from build123d import *

# Parameters (mm, degrees)
F0_W     = 63.5
F0_H     = 63.5
F1_DEPTH = 254
F2_R     = 30.48
F3_W     = 63.5
F3_H     = 33.02
F4_DEPTH = 38.1
F5_R     = 30.48


with BuildPart() as f1:
    # F0 (on Top) → F1 (new body)
    with BuildSketch(Plane.XY):
        with Locations((31.75, 31.75)):
            Rectangle(F0_W, F0_H)
    extrude(amount=F1_DEPTH)

    # F2
    f2_edges = [f1.edges().sort_by_distance(p)[0] for p in [
        (31.75, 0, 254),
    ]]
    fillet(f2_edges, radius=F2_R)

    # F3 (on face) → F4 (join)
    with BuildSketch(Plane.XY.offset(254)):
        with Locations((31.75, 46.99)):
            Rectangle(F3_W, F3_H)
    extrude(amount=F4_DEPTH)

    # F5
    f5_edges = [f1.edges().sort_by_distance(p)[0] for p in [
        (31.75, 63.5, 292.1),
    ]]
    fillet(f5_edges, radius=F5_R)


solid = f1.part
Can you work these out from the model? Positions are in its coordinate system, mm. A direction names the side the tool comes from. Coordinates: 2 decimals unless noted, no trailing zeros. Write each loop counter-clockwise with the first axis right and the second up, starting at its lowest first coordinate (ties: lowest second). Pieces come first, ordered by that corner, then holes. Notation, with made-up numbers: (70.25, 46.5) - (87.25, 46.5) arc R30 ccw to (87.25, 85.5) - close; hole circle Ø10 at (14.25, -21). An arc over 180 degrees is marked (long way). Return JSON: item names as keys, results as strings. Group by question number.
Item 1: Please list where these lines run through material, in increasing order: probe 1 along Z at (x, y) = (21.5, 29); probe 2 along Z at (x, y) = (59, 47); probe 3 along Y at (x, z) = (16, 269).
Item 2: If we section it at A-A (x = 33): Write out the boundary of the cut face in (y, z).
Item 3: If we section it at C-C (y = 49): Write out the boundary of the cut face in (x, z), then the cut area to 3 significant figures.
Item 4: Which directions (+Z, -Z, +X, -X, +Y, -Y) give clear straight access to the entire face, cutting with the end or side of a thin tool? Please do faces 1 (the face through (31, 30.48, 273)), 2 (the face through (32.19, 54.81, 282.93)).
Item 5: If we section it at B-B (z = 266.5): Write out the boundary of the cut face in (x, y), then the cut area to 3 significant figures.
Return value:
{
 "1": {"probe 1": "z = 0 to 253.96", "probe 2": "z = 0 to 288.7", "probe 3": "y = 30.48 to 62.59"},
 "2": {"outline": "(0, 0) - (63.5, 0) - (63.5, 261.62) arc R30.48 ccw to (33.02, 292.1) - (30.48, 292.1) - (30.48, 254) arc R30.48 ccw to (0, 223.52) - close"},
 "3": {"outline": "(0, 0) - (63.5, 0) - (63.5, 287.58) - (0, 287.58) - close", "area": "18,300 mm^2"},
 "4": {"face 1": "+Z, +X, -X, -Y", "face 2": "+Z, +X, -X, +Y"},
 "5": {"outline": "(0, 30.48) - (63.5, 30.48) - (63.5, 63.11) - (0, 63.11) - close", "area": "2,070 mm^2"}
}
